from build123d import *

# Parameters (mm, degrees)
F0_W     = 1370
F0_H     = 70
F1_DEPTH = 9
F2_W     = 1370
F2_H     = 50
F3_DEPTH = 9
F4_SIZE  = 10
F5_SIZE  = 5


with BuildPart() as f1:
    # F0 (on Front) → F1 (new body)
    with BuildSketch(Plane.XZ):
        Rectangle(F0_W, F0_H)
    extrude(amount=F1_DEPTH)

    # F2 (on face) → F3 (join)
    with BuildSketch(Plane.XZ.offset(9)):
        with Locations((0, 10)):
            Rectangle(F2_W, F2_H)
    extrude(amount=F3_DEPTH)

    # F4
    f4_edges = [f1.edges().sort_by_distance(p)[0] for p in [
        (685, -4.5, -35),
        (-685, -4.5, -35),
    ]]
    chamfer(f4_edges, length=F4_SIZE)

    # F5
    f5_edges = [f1.edges().sort_by_distance(p)[0] for p in [
        (0, 0, -35),
    ]]
    chamfer(f5_edges, length=F5_SIZE)


solid = f1.part
Can you work these out from the model? Positions are in its coordinate system, mm. Round coordinates to 2 decimals unless told otherwise and drop trailing zeros. Loops run counter-clockwise (first coordinate to the right, second up) from the corner with the lowest first, then second, coordinate; pieces in that order, holes last. Notation, with made-up numbers: (41.25, 73.5) - (48.25, 73.5) arc R23 ccw to (48.25, 89.5) - close; hole circle Ø8 at (10.5, 68.25). An arc over 180 degrees is marked (long way). Use CSV: the item, a comma, the result in double quotes. Start each with the question number.
1) Please list where these lines run through material, in increasing order: probe 1 along Z at (x, y) = (590, -10.5); probe 2 along Y at (x, z) = (273, -25.5); probe 3 along Z at (x, y) = (518, -0.75). Write a range as [from, to].
2) If we section it at B-B on y = -12: Write out the boundary of the cut face in (x, z).
3) For pin 1 Ø16 at (x, z) = (-56, -24) entering from -Y; pin 2 Ø2.5 at (x, y) = (129.5, -15.5) entering from -Z, each with a flat end and sliding along its axis, tell me the tip position at first contact or that it passes through.
4) If we section it at A-A on x = -598.5: Write out the boundary of the cut face in (y, z).
Geometry results:
1,probe 1,"z = [-15, 35]"
1,probe 2,"y = [-9, 0]"
1,probe 3,"z = [-30.75, 35]"
2,outline,"(-685, -15) - (685, -15) - (685, 35) - (-685, 35) - close"
3,pin 1,"stops at y = -9"
3,pin 2,"stops at z = -15"
4,outline,"(-18, -15) - (-9, -15) - (-9, -35) - (-5, -35) - (0, -30) - (0, 35) - (-18, 35) - close"
